```python
from build123d import *

# Parameters (mm, degrees)
F1_DEPTH = 80


with BuildPart() as f1:
    # F0 (on Front) → F1 (new body, symmetric)
    with BuildSketch(Plane.XZ):
        Polygon((-4.775, 10), (-10, 10), (-10, 4.775), (-8.325, 3.1), (-8.325, 5.5), (-6.684404, 5.5), (-3.75, 2.565596), (-3.75, 0), (-3.75, -2.565596), (-6.684404, -5.5), (-8.325, -5.5), (-8.325, -3.1), (-10, -4.775), (-10, -10), (-4.775, -10), (-3.1, -8.325), (-5.5, -8.325), (-5.5, -6.684404), (-2.565596, -3.75), (0, -3.75), (2.565596, -3.75), (5.5, -6.684404), (5.5, -8.325), (3.1, -8.325), (4.775, -10), (10, -10), (10, -4.775), (8.325, -3.1), (8.325, -5.5), (6.684404, -5.5), (3.75, -2.565596), (3.75, 0), (3.75, 2.565596), (6.684404, 5.5), (8.325, 5.5), (8.325, 3.1), (10, 4.775), (10, 10), (4.775, 10), (3.1, 8.325), (5.5, 8.325), (5.5, 6.684404), (2.565596, 3.75), (0, 3.75), (-2.565596, 3.75), (-5.5, 6.684404), (-5.5, 8.325), (-3.1, 8.325), align=None)
    extrude(amount=F1_DEPTH, both=True)


solid = f1.part
```
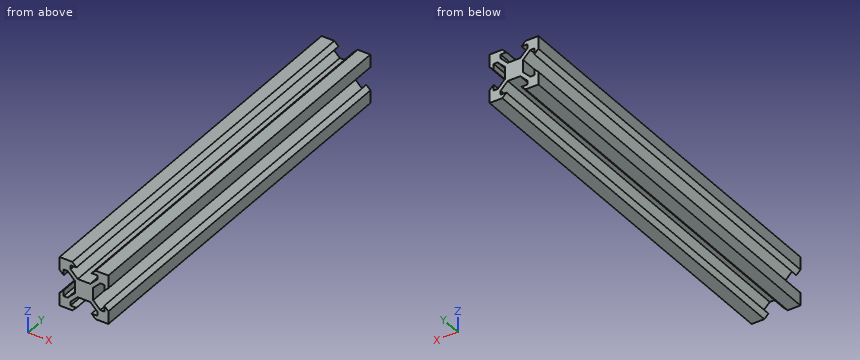
The listing builds one solid part. Answer for the finished solid, in the listing's coordinates (mm). Coordinates: 2 decimals unless noted, no trailing zeros. Loops run counter-clockwise (first coordinate to the right, second up) from the corner with the lowest first, then second, coordinate; pieces in that order, holes last. Notation, with made-up numbers: M 69.25,4.5 L 127.25,4.5 A15 cw 127.25,19.5 Z; hole C 50.5,-16.75 d2. An arc over 180 degrees is marked long. Answer as a JSON object with one key per item and string values. Group by question number.
Item 1: Consider L1, parallel to Z at x = -7.5, y = -26; L2, parallel to X at y = -23.5, z = 9 (3 decimals); L3, parallel to X at y = 22.5, z = 3.25 (3 decimals). Determine where each line is inside the solid, lowest interval first.
Item 2: Section A-A (x = -1.25) is taken. Write down the section's boundary in (y, z), and give its area (3 significant figures).
Item 3: Each of these flat-tipped pins is pushed along its axis until it touches: P1, Ø5, axis at x = 2, y = 63.5, coming from the -Z side (3 decimals); P2, Ø1, axis at x = 3, z = 7.5, coming from the -Y side; P3, Ø4, axis at x = 0.5, y = -33.5, coming from the +Z side; P4, Ø5.5, axis at y = 33, z = -1, coming from the +X side (3 decimals). Where does it stop, or does it pass through?
Solved:
{
 "1": {"L1": "z = -10 to -5.5, 5.5 to 10", "L2": "x = -10 to -3.775, 3.775 to 10", "L3": "x = -8.475 to -8.325, -4.434 to 4.434, 8.325 to 8.475"},
 "2": {"outline": "M -80,-3.75 L 80,-3.75 L 80,3.75 L -80,3.75 Z", "area": "1,200 mm2"},
 "3": {"P1": "stops at z = -9.725", "P2": "passes through", "P3": "stops at z = 3.75", "P4": "stops at x = 8.975"}
}
